The model under review builds one solid part; all positions refer to its coordinate system, in mm. Coordinates: 2 decimals unless noted, no trailing zeros. Loops run counter-clockwise (first coordinate to the right, second up) from the corner with the lowest first, then second, coordinate; pieces in that order, holes last. Notation, with made-up numbers: (-13, 68) - (-9, 68) arc R31 ccw to (-9, 92) - close; hole circle Ø2 at (16.25, -19). An arc over 180 degrees is marked (long way). Use a Markdown table: item, result. Add a question column.
1) To check wall thickness, follow L1, parallel to Z at x = 1.4, y = -1; L2, parallel to Z at x = 2.55, y = 4; L3, parallel to Y at x = 4.1, z = -66. State the ranges of each line that lie inside material, in increasing order. Write a range as [from, to].
2) Clearance check with a flat-ended pin moving along its axis: pin 1 (3 mm diameter, centred on x = 2.5, y = 7.5, fed in from -Z). State where the tip first meets the part, or that it passes through.
3) Add section A-A, the plane y = 2.75. Give the boundary of the cut face in (x, z).
4) Add section C-C, the plane y = 20.5. Give the boundary of the cut face in (x, z), and give its area (3 significant figures).
5) Add section B-B, the plane x = 1.1. Give the boundary of the cut face in (y, z).
6) Add section D-D, the plane z = -89. Give the boundary of the cut face in (x, y), and give its area (3 significant figures).
```python
from build123d import *

# Parameters (mm, degrees)
BOSS_EXTRUDE1_DEPTH = 5


with BuildPart() as part:
    # Sketch1 → Boss-Extrude1 (new body)
    with BuildSketch(Plane(origin=(0, 0, 0), x_dir=(0, 0, -1), z_dir=(1, 0, 0))):
        Polygon((0, 0), (0, 10), (9.902680687, 11.39173101), (9.206815183, 16.343071353), (14.158155526, 17.038936858), (14.854021031, 12.087596514), (54.464743781, 17.654520553), (53.768878276, 22.605860897), (58.72021862, 23.301726401), (59.416084124, 18.350386058), (99.026806874, 23.917310096), (99.026806874, 18.868172233), (90, 17.599537261), (90, 0), (80, 0), (80, -5), (75, -5), (75, 15.49142474), (15, 7.058974658), (15, -5), (10, -5), (10, 0), align=None)
    extrude(amount=BOSS_EXTRUDE1_DEPTH)


solid = part.part
```
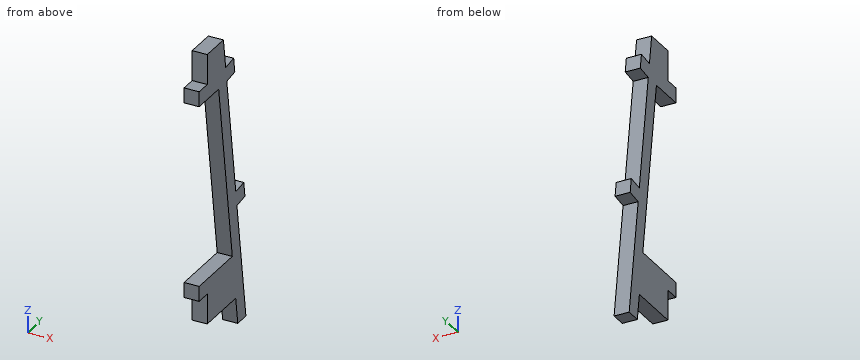
From the geometry:
| question | item | result |
|---|---|---|
| 1 | L1 | z = [-80, -75], [-15, -10] |
| 1 | L2 | z = [-90, -75], [-15, 0] |
| 1 | L3 | y = [14.23, 19.28] |
| 2 | pin 1 | stops at z = -90 |
| 3 | outline | (0, -90) - (5, -90) - (5, -75) - (0, -75) - close; (0, -15) - (5, -15) - (5, 0) - (0, 0) - close |
| 4 | outline | (0, -99.03) - (5, -99.03) - (5, -74.71) - (0, -74.71) - close; (0, -59.11) - (5, -59.11) - (5, -54.06) - (0, -54.06) - close |
| 4 | area | 147 mm^2 |
| 5 | outline | (-5, -80) - (0, -80) - (0, -90) - (17.6, -90) - (18.87, -99.03) - (23.92, -99.03) - (18.35, -59.42) - (23.3, -58.72) - (22.61, -53.77) - (17.65, -54.46) - (12.09, -14.85) - (17.04, -14.16) - (16.34, -9.21) - (11.39, -9.9) - (10, 0) - (0, 0) - (0, -10) - (-5, -10) - (-5, -15) - (7.06, -15) - (15.49, -75) - (-5, -75) - close |
| 6 | outline | (0, 0) - (5, 0) - (5, 22.51) - (0, 22.51) - close |
| 6 | area | 113 mm^2 |
